Geometry check sheet. Reference: the model listing, model coordinates, mm. Round coordinates to 2 decimals unless told otherwise and drop trailing zeros. Order: outer loops, then holes, each group sorted by start corner. A loop starts at its lowest first (then second) coordinate and runs counter-clockwise, first axis right, second up. Notation, with made-up numbers: (25.5, 18) - (78.5, 18) arc R13 ccw to (78.5, 39) - close; hole circle Ø7 at (11.5, -40). An arc over 180 degrees is marked (long way). Use a Markdown table: item, result. Add a question column.
(1) Section check A-A on z = -95.25. Record the boundary of the cut face in (x, y) (3 decimals), then the cut area to 3 significant figures.
(2) Section check C-C on y = 1.2. Give the number of separate pieces and of enclosed holes in the cut face, then the cut area to 3 significant figures.
(3) Section check B-B on z = -57.15. Record the boundary of the cut face in (x, y) (3 decimals), then the cut area to 3 significant figures.
(4) Thickness scan on line 1 along X through (y, z) = (1.35, -95); line 2 along X through (y, z) = (1, -95.25); line 3 along X through (y, z) = (1.5, -36.5) (3 decimals). Record the ranges inside material, lowest first. Write a range as [from, to].
(5) Gauge pin test, flat ends, axial feed: P1, Ø3.5, axis at x = 9.525, z = -12.7, coming from the -Y side; P2, Ø1.6, axis at y = 2, z = -8.5, coming from the -X side (3 decimals); P3, Ø1.6, axis at x = 145, y = 1, coming from the +Z side. Record the tip position at first contact, or that the pin passes through.
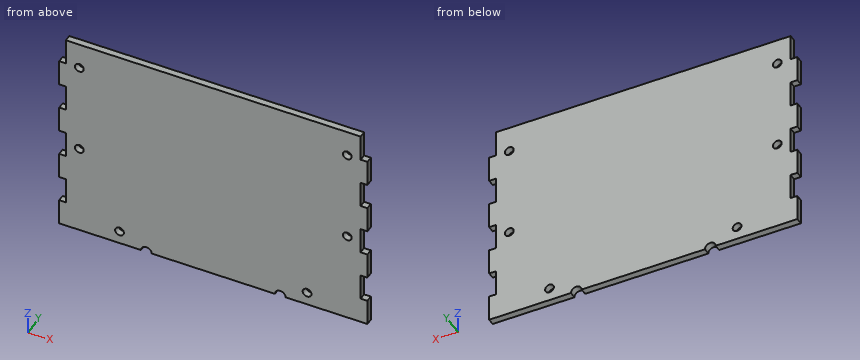
```python
from build123d import *

# Parameters (mm, degrees)
SKETCH2_R           = 2.0828
BOSS_EXTRUDE1_DEPTH = 3.175


with BuildPart() as part:
    # Sketch2 → Boss-Extrude1 (new body)
    with BuildSketch(Plane(origin=(0, 0, 0), x_dir=(1, 0, 0), z_dir=(0, 1, 0))):
        with BuildLine():
            Line((3.175, 0), (3.175, 12.7))
            Line((3.175, 12.7), (0, 12.7))
            Line((0, 12.7), (0, 25.4))
            Line((0, 25.4), (3.175, 25.4))
            Line((3.175, 25.4), (3.175, 38.1))
            Line((3.175, 38.1), (0, 38.1))
            Line((0, 38.1), (0, 50.8))
            Line((0, 50.8), (3.175, 50.8))
            Line((3.175, 50.8), (3.175, 63.5))
            Line((3.175, 63.5), (0, 63.5))
            Line((0, 63.5), (0, 76.2))
            Line((0, 76.2), (3.175, 76.2))
            Line((3.175, 76.2), (3.175, 88.9))
            Line((3.175, 88.9), (0, 88.9))
            Line((0, 88.9), (0, 101.6))
            Line((0, 101.6), (3.175, 101.6))
            Line((3.175, 101.6), (38.735, 101.6))
            ThreePointArc((38.735, 101.6), (41.275, 99.06), (43.815, 101.6))
            Line((43.815, 101.6), (102.235, 101.6))
            ThreePointArc((102.235, 101.6), (104.775, 99.06), (107.315, 101.6))
            Line((107.315, 101.6), (142.875, 101.6))
            Line((142.875, 101.6), (146.05, 101.6))
            Line((146.05, 101.6), (146.05, 88.9))
            Line((146.05, 88.9), (142.875, 88.9))
            Line((142.875, 88.9), (142.875, 76.2))
            Line((142.875, 76.2), (146.05, 76.2))
            Line((146.05, 76.2), (146.05, 63.5))
            Line((146.05, 63.5), (142.875, 63.5))
            Line((142.875, 63.5), (142.875, 50.8))
            Line((142.875, 50.8), (146.05, 50.8))
            Line((146.05, 50.8), (146.05, 38.1))
            Line((146.05, 38.1), (142.875, 38.1))
            Line((142.875, 38.1), (142.875, 25.4))
            Line((142.875, 25.4), (146.05, 25.4))
            Line((146.05, 25.4), (146.05, 12.7))
            Line((146.05, 12.7), (142.875, 12.7))
            Line((142.875, 12.7), (142.875, 0))
            Line((142.875, 0), (3.175, 0))
        make_face()
        with Locations(Location((136.525, 57.15, 0), (0, 0, 90))):
            Circle(SKETCH2_R, mode=Mode.SUBTRACT)
        with Locations(Location((9.525, 12.7, 0), (0, 0, 270))):
            Circle(SKETCH2_R, mode=Mode.SUBTRACT)
        with Locations(Location((9.525, 57.15, 0), (0, 0, 270))):
            Circle(SKETCH2_R, mode=Mode.SUBTRACT)
        with Locations(Location((136.525, 12.7, 0), (0, 0, 90))):
            Circle(SKETCH2_R, mode=Mode.SUBTRACT)
        with Locations(Location((28.575, 95.25, 0), (0, 0, 270))):
            Circle(SKETCH2_R, mode=Mode.SUBTRACT)
        with Locations(Location((117.475, 95.25, 0), (0, 0, 90))):
            Circle(SKETCH2_R, mode=Mode.SUBTRACT)
    extrude(amount=BOSS_EXTRUDE1_DEPTH)


solid = part.part
```
Check sheet entries:
| question | item | result |
|---|---|---|
| 1 | outline | (0, 0) - (26.492, 0) - (26.492, 3.175) - (0, 3.175) - close; (30.658, 0) - (115.392, 0) - (115.392, 3.175) - (30.658, 3.175) - close; (119.558, 0) - (146.05, 0) - (146.05, 3.175) - (119.558, 3.175) - close |
| 1 | area | 437 mm2 |
| 2 | separate pieces | 1 |
| 2 | enclosed holes | 6 |
| 2 | area | 14,400 mm2 |
| 3 | outline | (3.175, 0) - (7.442, 0) - (7.442, 3.175) - (3.175, 3.175) - close; (11.608, 0) - (134.442, 0) - (134.442, 3.175) - (11.608, 3.175) - close; (138.608, 0) - (142.875, 0) - (142.875, 3.175) - (138.608, 3.175) - close |
| 3 | area | 417 mm2 |
| 4 | line 1 | x = [0, 26.51], [30.64, 115.41], [119.54, 146.05] |
| 4 | line 2 | x = [0, 26.49], [30.66, 115.39], [119.56, 146.05] |
| 4 | line 3 | x = [3.175, 142.875] |
| 5 | P1 | passes through |
| 5 | P2 | stops at x = 3.175 |
| 5 | P3 | stops at z = -12.7 |
